Check sheet for the modelled part. Datum: model origin and axes. Units: mm. Round coordinates to 2 decimals unless told otherwise and drop trailing zeros. Write each loop counter-clockwise with the first axis right and the second up, starting at its lowest first coordinate (ties: lowest second). Pieces come first, ordered by that corner, then holes.
Item 1: Depth check by flat-ended pin: pin 1 (10 mm diameter, centred on x = 4, y = 1.5, fed in from +Z); pin 2 (1.5 mm diameter, centred on y = 3, z = 8, fed in from -X); pin 3 (4 mm diameter, centred on y = 2.5, z = 12, fed in from +X); pin 4 (2 mm diameter, centred on x = 3.5, z = 5, fed in from -Y). Enter the tip coordinate at first touch or a pass-through.
Item 2: Section check A-A, the plane z = 9.25. Record the cut outline in (x, y) (3 decimals).
Item 3: Material ranges on line 1 along Y through (x, z) = (0, 9); line 2 along X through (y, z) = (0, 6.75); line 3 along X through (y, z) = (-12, 8.5), recorded low to high.
Item 4: Release check for a two-part mould opening along X. For faces 1 (the flat face through (-16, 6, 2.777)), 2 (the cylindrical face through (-2.76, -18.26, 7.91)), 3 (the cylindrical face through (12.84, -4.16, 7.89)) record: pulls with the +X half, pulls with the -X half, needs draft (parallel to the pull), parting line crosses it, or undercut.
from build123d import *

# Parameters (mm, degrees)
F0_W = 4.572
F0_H = 10.16
F2_R = 2.54
F3_R = 1.27


with BuildPart() as f1:
    # F0 (on Front) → F1 (revolve)
    with BuildSketch(Plane.XZ):
        with Locations((15.7638760562, 7.8567868348)):
            Rectangle(F0_W, F0_H)
    revolve(axis=Axis((-0.3651239438, 0, 7.8567868348), (0, 0, -1)))

    # F2
    f2_edges = [f1.edges().sort_by_distance(p)[0] for p in [
        (-14.208124, 0, 12.936787),
        (-14.208124, 0, 2.776787),
    ]]
    fillet(f2_edges, radius=F2_R)

    # F3
    f3_edges = [f1.edges().sort_by_distance(p)[0] for p in [
        (-18.780124, 0, 12.936787),
        (-18.780124, 0, 2.776787),
    ]]
    fillet(f3_edges, radius=F3_R)


solid = f1.part
Values found:
1. pin 1: passes through
1. pin 2: stops at x = -18.64
1. pin 3: stops at x = 18.04
1. pin 4: stops at y = -18.19
2. outline: circle Ø36.83 at (-0.365, 0); hole circle Ø27.686 at (-0.365, 0)
3. line 1: y = -18.41 to -13.84, 13.84 to 18.41
3. line 2: x = -18.78 to -14.21, 13.48 to 18.05
3. line 3: x = -14.33 to -7.27, 6.54 to 13.6
4. face 1: needs draft
4. face 2: parting line crosses it
4. face 3: undercut
